Geometry: final body of the model. Coordinates: model frame, mm. A direction names the side the tool comes from. Round coordinates to 2 decimals unless told otherwise and drop trailing zeros. Loops run counter-clockwise (first coordinate to the right, second up) from the corner with the lowest first, then second, coordinate; pieces in that order, holes last. Notation, with made-up numbers: M -10.5,34 L 21.5,34 A8 ccw 21.5,49 Z; hole C -33.5,51 d11. An arc over 180 degrees is marked long. Answer as a JSON object with one key per item and string values.
Autodesk Inventor part; units mm, degrees
ref_plane "YZ Plane" through (0, 0, 0) normal (1, 0, 0) x (0, 1, 0)
ref_plane "XZ Plane" through (0, 0, 0) normal (0, 1, 0) x (-1, 0, 0)
ref_plane "XY Plane" through (0, 0, 0) normal (0, 0, 1) x (1, 0, 0)
sketch "Sketch1" plane through (0, 0, 0) normal (0, 0, 1) x (1, 0, 0)
  line L0 (-15, -15) -> (15, -15)
  line L1 (15, -15) -> (15, 15)
  line L2 (15, 15) -> (-15, 15)
  line L3 (-15, 15) -> (-15, -15)
  line L4 (-15, -15) -> (15, 15) construction
  line L5 (15, -15) -> (-15, 15) construction
  line L6 (0, -10) -> (0, 10)
  line L7 (-10, 0) -> (10, 0)
  circle A0 centre (-10, 0) radius 2.55
  circle A1 centre (0, 10) radius 2.55
  circle A2 centre (10, 0) radius 2.55
  circle A3 centre (0, -10) radius 2.55
  line L8 (-15, -15) -> (15, -15)
  line L9 (15, -15) -> (15, -18)
  line L10 (15, -18) -> (-15, -18)
  line L11 (-15, -18) -> (-15, -15)
  point P0 (0, 0)
  dimension "d0" = 30
  dimension "d1" = 30
  dimension "d2" = 20
  dimension "d3" = 20
  dimension "d4" = 5.1
  dimension "d5" = 5.1
  dimension "d6" = 5.1
  dimension "d7" = 5.1
  dimension "d8" = 3
extrude "Extrusion1" add sketch "Sketch1" along normal blind 3
extrude "Extrusion2" add sketch "Sketch1" against normal blind 40 contours L0 L9 L10 L11
sketch "Sketch2" plane through (-15, -15, 0) normal (0, 1, 0) x (1, 0, 0)
  line L0 (0, 0) -> (0, -3)
  line L1 (30, 0) -> (30, 40)
  line L2 (0, 0) -> (30, 0)
  line L3 (30, 0) -> (15, 0)
  line L4 (15, 0) -> (15, 22.896)
  circle A0 centre (15, 22.896) radius 5.1
  circle A1 centre (15, 22.896) radius 8
  circle A2 centre (15, 14.896) radius 1.75
  circle A3 centre (23, 22.896) radius 1.75
  circle A4 centre (15, 30.896) radius 1.75
  circle A5 centre (7, 22.896) radius 1.75
  point P0 (13.2605, 30.7046)
  point P1 (16.7395, 30.7046)
  dimension "d15" = 16
  dimension "d13" = 22.896
  dimension "d14" = 10.2
  dimension "d16" = 3.5
  dimension "d19" = 360
extrude "Extrusion3" cut sketch "Sketch2" against normal blind 40 contours A2 A1 L4 | L4 A1 A2 | A1 A2 L4 | L4 A2 A1 | A0 | A5 A1 | A1 A5 | A3 A1 | A1 A3 | A4 A1 | A1 A4
properties part number "Leadnut Attachment"
1) Section query B-B (z = 0.5). Return the cut outline in (x, y), and give its area (3 significant figures).
Results:
{"outline": "M -15,-18 L 15,-18 L 15,15 L -15,15 Z; hole C -10,0 d5.1; hole C 0,-10 d5.1; hole C 0,10 d5.1; hole C 10,0 d5.1", "area": "908 mm2"}
2) Section query C-C (x = 0). Return the cut outline in (y, z), and give its area (3 significant figures).
Results:
{"outline": "M -18,-40 L -15,-40 L -15,-32.65 L -18,-32.65 Z; M -18,-29.15 L -15,-29.15 L -15,-28 L -18,-28 Z; M -18,-17.8 L -15,-17.8 L -15,-16.65 L -18,-16.65 Z; M -18,-13.15 L -15,-13.15 L -15,0 L -12.55,0 L -12.55,3 L -18,3 Z; M -7.45,0 L 7.45,0 L 7.45,3 L -7.45,3 Z; M 12.55,0 L 15,0 L 15,3 L 12.55,3 Z", "area": "137 mm2"}
3) Ray query, line 1 (Y direction, x = 0, z = 2.1); line 2 (X direction, y = 10, z = 2.45); line 3 (Y direction, x = -10, z = 1.7). Return the intervals inside material, ascending.
Results:
{"line 1": "-18 to -12.55, -7.45 to 7.45, 12.55 to 15", "line 2": "-15 to -2.55, 2.55 to 15", "line 3": "-18 to -2.55, 2.55 to 15"}
4) Section query D-D (y = 0). Return the cut outline in (x, z), and give its area (3 significant figures).
Results:
{"outline": "M -15,0 L -12.55,0 L -12.55,3 L -15,3 Z; M -7.45,0 L 7.45,0 L 7.45,3 L -7.45,3 Z; M 12.55,0 L 15,0 L 15,3 L 12.55,3 Z", "area": "59.4 mm2"}
5) Pin query (flat end, axial travel): P1, Ø6.5, axis at x = 10, y = 0, coming from the +Z side; P2, Ø9, axis at x = 0, z = -22.896, coming from the -Y side; P3, Ø6.5, axis at x = -10, y = 0, coming from the -Z side; P4, Ø8, axis at x = -0.5, z = -14, coming from the +Y side. Return the tip coordinate at first contact, or that it passes through.
Results:
{"P1": "z = 3", "P2": "through", "P3": "z = 0", "P4": "y = -15"}
6) Reachability of faces 1 (the flat face through (3, -15, -15)), 2 (the cylindrical face through (0.94, -16.48, -32.37)) from +Z, -Z, +X, -X, +Y, -Y: full face, straight path, thin tool, end or side. Return the list, or none.
Results:
{"face 1": "-Z, +X, -X, +Y", "face 2": "+Y, -Y"}
7) Pull-direction query (Z, two-part tool) for faces 3 (the flat face through (0, 15, 1)), 4 (the flat face through (0, 0, 0)), 5 (the cylindrical face through (8.94, -16.48, -24.37)), 6 (the flat face through (0, -1, 3)); classes: +Z half, -Z half, draft (parallel to the pull), parting line (faces both ways), or undercut.
Results:
{"face 3": "draft", "face 4": "-Z half", "face 5": "undercut", "face 6": "+Z half"}
8) Section query A-A (y = -10). Return the cut outline in (x, z), and give its area (3 significant figures).
Results:
{"outline": "M -15,0 L -2.55,0 L -2.55,3 L -15,3 Z; M 2.55,0 L 15,0 L 15,3 L 2.55,3 Z", "area": "74.7 mm2"}
